from build123d import *

# Parameters (mm, degrees)
CROQUIS1_R                 = 22.5
SALIENTE_EXTRUIR1_DEPTH    = 3
CROQUIS2_R                 = 12.5
SALIENTE_EXTRUIR2_DEPTH    = 10
CROQUIS3_R                 = 5
CORTAR_EXTRUIR1_DEPTH      = 35.372954485
CROQUIS4_R                 = 2
CORTAR_EXTRUIR2_DEPTH      = 34.35416016
CORTAR_EXTRUIR3_DEPTH      = 35.372954485
CORTAR_EXTRUIR3_DEPTH_BACK = 35.372954485
CROQUIS5_R                 = 2
CORTAR_EXTRUIR4_DEPTH      = 35.372954522
CORTAR_EXTRUIR4_DEPTH_BACK = 35.372954522
CROQUIS6_R                 = 2


with BuildPart() as part:
    # Croquis1 → Saliente-Extruir1 (new body)
    with BuildSketch(Plane.XY):
        Circle(CROQUIS1_R)
    extrude(amount=SALIENTE_EXTRUIR1_DEPTH)

    # Croquis2 → Saliente-Extruir2 (add)
    with BuildSketch(Plane.XY.offset(3)):
        Circle(CROQUIS2_R)
    extrude(amount=SALIENTE_EXTRUIR2_DEPTH)

    # Croquis3 → Cortar-Extruir1 (cut, through all)
    with BuildSketch(Plane.XY.offset(13)):
        Circle(CROQUIS3_R)
    extrude(amount=-CORTAR_EXTRUIR1_DEPTH, mode=Mode.SUBTRACT)

    # Croquis4 → Cortar-Extruir2 (cut, through all)
    with BuildSketch(Plane.XY.offset(3)):
        with Locations((-4.962538649, 15.414885677)):
            Circle(CROQUIS4_R)
        with Locations((15.414885677, 4.962538649)):
            Circle(CROQUIS4_R)
        with Locations((4.962538649, -15.414885677)):
            Circle(CROQUIS4_R)
        with Locations((-15.414885677, -4.962538649)):
            Circle(CROQUIS4_R)
    extrude(amount=-CORTAR_EXTRUIR2_DEPTH, mode=Mode.SUBTRACT)

    # Croquis5 → Cortar-Extruir3 (cut, two sides: drawn at the far end of the back side and taken through both)
    with BuildSketch(Plane(origin=(0, 0, 0), x_dir=(0, 0, -1), z_dir=(1, 0, 0)).offset(-CORTAR_EXTRUIR3_DEPTH_BACK)):
        with Locations((-8, 0)):
            Circle(CROQUIS5_R)
    extrude(amount=CORTAR_EXTRUIR3_DEPTH + CORTAR_EXTRUIR3_DEPTH_BACK, mode=Mode.SUBTRACT)

    # Croquis6 → Cortar-Extruir4 (cut, two sides: drawn at the far end of the back side and taken through both)
    with BuildSketch(Plane(origin=(0, 0, 0), x_dir=(1, 0, 0), z_dir=(0, 1, 0)).offset(-CORTAR_EXTRUIR4_DEPTH_BACK)):
        with Locations(Location((0, -8.215337569, 0), (0, 0, 270))):
            Circle(CROQUIS6_R)
    extrude(amount=CORTAR_EXTRUIR4_DEPTH + CORTAR_EXTRUIR4_DEPTH_BACK, mode=Mode.SUBTRACT)


solid = part.part
Geometry check sheet. Reference: the model listing, model coordinates, mm. A direction names the side the tool comes from. Round coordinates to 2 decimals unless told otherwise and drop trailing zeros. Order: outer loops, then holes, each group sorted by start corner. A loop starts at its lowest first (then second) coordinate and runs counter-clockwise, first axis right, second up. Notation, with made-up numbers: M 34,82.5 L 93,82.5 A23 cw 93,108.5 Z; hole C 79,-18.5 d8. An arc over 180 degrees is marked long. Answer in a Markdown table with one row per item.
(1) Go/stop test with flat-tipped pins: P1, Ø5, axis at x = -4.96, y = 15.41, coming from the +Z side; P2, Ø1, axis at x = 8, y = 12, coming from the -Z side; P3, Ø2, axis at y = 11, z = 4.5, coming from the +X side; P4, Ø5, axis at x = 0, z = 8.22, coming from the -Y side. Record where each tip stops, or that it passes through.
Responses:
| item | result |
|---|---|
| P1 | stops at z = 3 |
| P2 | stops at z = 0 |
| P3 | stops at x = 7.5 |
| P4 | stops at y = -12.5 |
(2) Sectioned sample at D-D, the plane y = 9. Record the cut outline in (x, z).
Responses:
| item | result |
|---|---|
| outline | M -20.62,0 L 20.62,0 L 20.62,3 L 8.67,3 L 8.67,13 L -8.67,13 L -8.67,3 L -20.62,3 Z; hole C 0,8.22 d4 |
(3) Sectioned sample at C-C, the plane z = 11. Record the cut outline in (x, y), and give its area (3 significant figures).
Responses:
| item | result |
|---|---|
| outline | C 0,0 d25; hole C 0,0 d10 |
| area | 412 mm² |
(4) Scan lines: probe 1 along Z at (x, y) = (0, -10); probe 2 along Z at (x, y) = (10.75, 0); probe 3 along Z at (x, y) = (-10, 19.5). Record each from-to range of solid material in increasing order. Write a range as from..to.
Responses:
| item | result |
|---|---|
| probe 1 | z = 0..6.22, 10.22..13 |
| probe 2 | z = 0..6, 10..13 |
| probe 3 | z = 0..3 |
(5) Draft check along Y on faces 1 (the face through (-0.77, -8.6, 10.06)), 2 (the face through (10.382, -19.961, 1.479)), 3 (the face through (8.486, -0.766, 6.153)). Enter one of: released by +Y, released by -Y, zero draft, split by the parting line, or undercut.
Responses:
| item | result |
|---|---|
| face 1 | zero draft |
| face 2 | split by the parting line |
| face 3 | undercut |
(6) Sectioned sample at A-A, the plane y = 0. Record the cut outline in (x, z), and give its area (3 significant figures).
Responses:
| item | result |
|---|---|
| outline | M -22.5,0 L -5,0 L -5,6 L -12.5,6 L -12.5,3 L -22.5,3 Z; M -12.5,10 L -5,10 L -5,13 L -12.5,13 Z; M 5,0 L 22.5,0 L 22.5,3 L 12.5,3 L 12.5,6 L 5,6 Z; M 5,10 L 12.5,10 L 12.5,13 L 5,13 Z |
| area | 195 mm² |
(7) Sectioned sample at B-B, the plane x = 0. Record the cut outline in (y, z).
Responses:
| item | result |
|---|---|
| outline | M -22.5,0 L -5,0 L -5,6.22 L -12.5,6.22 L -12.5,3 L -22.5,3 Z; M -12.5,10.22 L -5,10.22 L -5,13 L -12.5,13 Z; M 5,0 L 22.5,0 L 22.5,3 L 12.5,3 L 12.5,6.22 L 5,6.22 Z; M 5,10.22 L 12.5,10.22 L 12.5,13 L 5,13 Z |
(8) Tool access check on faces 4 (the face through (11.547, -4.788, 7.93)), 5 (the face through (5.885, -17.189, 1.521)). Record the directions out of +Z, -Z, +X, -X, +Y, -Y that give a thin tool (end or side, any length) a straight path to the whole face; none if there is none.
Responses:
| item | result |
|---|---|
| face 4 | +Z |
| face 5 | +Z, -Z |
